Input: part model. Units: mm. Frame: model coordinates. Round coordinates to 2 decimals unless told otherwise and drop trailing zeros. Order: outer loops, then holes, each group sorted by start corner. A loop starts at its lowest first (then second) coordinate and runs counter-clockwise, first axis right, second up.
Item 1: Cut plane B-B on y = -18. Output: boundary loops of the cut face in (x, z), then the cut area to 3 significant figures.
Item 2: Mould query, pull axis X, two halves, no side actions, for faces 1 (the cylindrical face through (-6, 0, 0)), 2 (the cylindrical face through (120, 0, 0)), 3 (the flat face through (49, 20, 0)). Classes: released by +X, released by -X, zero draft, split by the parting line, or undercut.
Item 3: Line query: L1, parallel to Y at x = 94.5, z = -0.1; L2, parallel to Y at x = 24.5, z = -0.25; L3, parallel to X at y = 8, z = -1.35. Output: solid intervals per line, ascending.
Item 4: First-contact query: pin 1 (2 mm diameter, centred on y = -10.5, z = -1, fed in from +X); pin 2 (2 mm diameter, centred on y = 10.5, z = -2, fed in from -X). Flat tips, straight axial feed; report the tip coordinate or a pass-through.
Item 5: Cut plane A-A on z = 0.1. Give the number of separate pieces and of enclosed holes in the cut face, then the cut area to 3 significant figures.
```python
from build123d import *

# Parameters (mm, degrees)
SKETCH1_R           = 6
SKETCH1_R_2         = 1
SKETCH1_R_3         = 11
SKETCH1_R_4         = 1.05
BOSS_EXTRUDE1_DEPTH = 2.5


with BuildPart() as part:
    # Sketch1 → Boss-Extrude1 (new, symmetric)
    with BuildSketch(Plane.XY):
        with BuildLine():
            Line((0, 20), (100, 20))
            ThreePointArc((100, 20), (120, 0), (100, -20))
            Line((100, -20), (0, -20))
            ThreePointArc((0, -20), (-20, 0), (0, 20))
        make_face()
        Circle(SKETCH1_R, mode=Mode.SUBTRACT)
        with Locations((9.5, 0)):
            Circle(SKETCH1_R_2, mode=Mode.SUBTRACT)
        with Locations((14.5, 0)):
            Circle(SKETCH1_R_2, mode=Mode.SUBTRACT)
        with Locations((19.5, 0)):
            Circle(SKETCH1_R_2, mode=Mode.SUBTRACT)
        with Locations((24.5, 0)):
            Circle(SKETCH1_R_2, mode=Mode.SUBTRACT)
        with Locations((29.5, 0)):
            Circle(SKETCH1_R_2, mode=Mode.SUBTRACT)
        with Locations((34.5, 0)):
            Circle(SKETCH1_R_2, mode=Mode.SUBTRACT)
        with Locations((39.5, 0)):
            Circle(SKETCH1_R_2, mode=Mode.SUBTRACT)
        with Locations((100, 0)):
            Circle(SKETCH1_R_3, mode=Mode.SUBTRACT)
        with Locations((0, 12)):
            Circle(SKETCH1_R_4, mode=Mode.SUBTRACT)
        with Locations((8.485281374, 8.485281374)):
            Circle(SKETCH1_R_4, mode=Mode.SUBTRACT)
        with Locations((12, 0)):
            Circle(SKETCH1_R_4, mode=Mode.SUBTRACT)
        with Locations((8.485281374, -8.485281374)):
            Circle(SKETCH1_R_4, mode=Mode.SUBTRACT)
        with Locations((0, -12)):
            Circle(SKETCH1_R_4, mode=Mode.SUBTRACT)
        with Locations((-8.485281374, -8.485281374)):
            Circle(SKETCH1_R_4, mode=Mode.SUBTRACT)
        with Locations((-12, 0)):
            Circle(SKETCH1_R_4, mode=Mode.SUBTRACT)
        with Locations((-8.485281374, 8.485281374)):
            Circle(SKETCH1_R_4, mode=Mode.SUBTRACT)
    extrude(amount=BOSS_EXTRUDE1_DEPTH, both=True)


solid = part.part
```
From the geometry:
1. outline: (-8.72, -2.5) - (108.72, -2.5) - (108.72, 2.5) - (-8.72, 2.5) - close
1. area: 587 mm2
2. face 1: undercut
2. face 2: released by +X
2. face 3: zero draft
3. L1: y = -20 to -9.53, 9.53 to 20
3. L2: y = -20 to -1, 1 to 20
3. L3: x = -18.33 to -9.42, -7.55 to 7.55, 9.42 to 92.45, 107.55 to 118.33
4. pin 1: stops at x = 117.6
4. pin 2: stops at x = -17.6
5. separate pieces: 1
5. enclosed holes: 17
5. area: 4,710 mm2
